Could you check a few things on this model? Use its own coordinates, in mm. Face numbers are marked on the shaded views. A direction names the side the tool comes from. Round coordinates to 2 decimals unless told otherwise and drop trailing zeros. Loops run counter-clockwise (first coordinate to the right, second up) from the corner with the lowest first, then second, coordinate; pieces in that order, holes last. Notation, with made-up numbers: (45.5, 4.25) -> (94.5, 4.25) arc R22 cw to (94.5, 21.25) -> close; hole circle Ø5 at (-20.75, -35). An arc over 180 degrees is marked (long way). One line per item, written item: value.
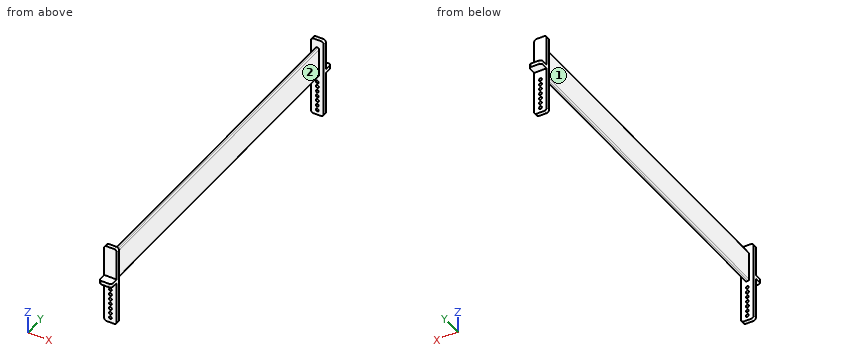
```python
from build123d import *

# Parameters (mm, degrees)
F0_W     = 15.875
F0_H     = 101.6
F4_DEPTH = 4.7625
F2_W     = 15.875
F2_H     = 4.7625
F5_DEPTH = 10.795
F1_W     = 4.7625
F1_H     = 38.1
F6_DEPTH = 431.8
F7_START = 431.8
F7_DEPTH = 4.7625
F8_START = 436.5625
F8_DEPTH = 10.795
F3_R     = 1.905
F3_R_2   = 1.8018515142
F3_R_3   = 1.8092820601
F9_DEPTH = 447.3585
F11_R    = 1.5875
F12_R    = 3.175


with BuildPart() as f4:
    # F0 (on Front) → F4 (new body)
    with BuildSketch(Plane.XZ):
        Rectangle(F0_W, F0_H)
    extrude(amount=F4_DEPTH)

    # F2 (on Front) → F5 (join)
    with BuildSketch(Plane.XZ):
        with Locations((0, 8.28675)):
            Rectangle(F2_W, F2_H)
    extrude(amount=-F5_DEPTH)

    # F1 (on Front) → F6 (join)
    with BuildSketch(Plane.XZ):
        with Locations((0, 21.2725)):
            Rectangle(F1_W, F1_H)
    extrude(amount=F6_DEPTH)

    # F0 (on Front) → F7 (join)
    with BuildSketch(Plane.XZ.offset(F7_START)):
        Rectangle(F0_W, F0_H)
    extrude(amount=F7_DEPTH)

    # F2 (on Front) → F8 (join)
    with BuildSketch(Plane.XZ.offset(F8_START)):
        with Locations((0, 8.28675)):
            Rectangle(F2_W, F2_H)
    extrude(amount=F8_DEPTH)

    # F3 (on Front) → F9 (cut, through all)
    with BuildSketch(Plane.XZ):
        with Locations((0, -31.75)):
            Circle(F3_R)
        with Locations((0, -38.1)):
            Circle(F3_R_2)
        with Locations((0, -44.45)):
            Circle(F3_R_3)
        with Locations((0, -12.7)):
            Circle(F3_R)
        with Locations((0, -19.05)):
            Circle(F3_R_2)
        with Locations((0, -25.4)):
            Circle(F3_R_3)
        with Locations((0, -6.35)):
            Circle(F3_R_2)
    extrude(amount=F9_DEPTH, mode=Mode.SUBTRACT)

    # F11
    f11_edges = [f4.edges().sort_by_distance(p)[0] for p in [
        (-2.38125, -218.28125, 40.3225),
        (2.38125, -218.28125, 40.3225),
        (2.38125, -218.28125, 2.2225),
        (-2.38125, -218.28125, 2.2225),
    ]]
    fillet(f11_edges, radius=F11_R)

    # F12
    f12_edges = [f4.edges().sort_by_distance(p)[0] for p in [
        (7.9375, -434.18125, 50.8),
        (-7.9375, -434.18125, 50.8),
        (7.9375, -434.18125, -50.8),
        (-7.9375, -434.18125, -50.8),
        (-7.9375, -447.3575, 8.28675),
        (7.9375, -447.3575, 8.28675),
        (7.9375, -2.38125, 50.8),
        (-7.9375, -2.38125, 50.8),
        (7.9375, -2.38125, -50.8),
        (-7.9375, -2.38125, -50.8),
        (-7.9375, 10.795, 8.28675),
        (7.9375, 10.795, 8.28675),
    ]]
    fillet(f12_edges, radius=F12_R)


solid = f4.part
```
(1) On a 3-axis mill with a long thin cutter (end or side, diameter ignored), from which of +Z, -Z, +X, -X, +Y, -Y can I reach the whole of each face in a straight line? I mean the marked faces 1 and 2. Say none if no direction works.
Results below:
face 1: +Z, -Z, -X
face 2: +Z, -Z, +X
(2) Please list where these lines run through material, in increasing order: L1, parallel to X at y = -433, z = -44; L2, parallel to Y at x = 4, z = 37; L3, parallel to Y at x = 5.25, z = 6.5.
Results below:
L1: x = -7.94 to -1.75, 1.75 to 7.94
L2: y = -436.56 to -431.8, -4.76 to 0
L3: y = -447.32 to -431.8, -4.76 to 10.76
(3) Imagine slicing it at A-A on y = -144.5. Write out the boundary of the cut face in (x, z) (1 decimal).
Results below:
outline: (-2.4, 3.8) arc R1.6 ccw to (-0.8, 2.2) -> (0.8, 2.2) arc R1.6 ccw to (2.4, 3.8) -> (2.4, 38.7) arc R1.6 ccw to (0.8, 40.3) -> (-0.8, 40.3) arc R1.6 ccw to (-2.4, 38.7) -> close
(4) For pin 1 Ø2 at (x, z) = (0, -6.35) entering from +Y; pin 2 Ø4.5 at (x, z) = (0, -44.45) entering from +Y; pin 3 Ø8 at (y, z) = (-267, 18.5) entering from +X; pin 4 Ø2 at (x, y) = (2, -331.5) entering from +Z, each with a flat end and sliding along its axis, tell me the tip position at first contact or that it passes through.
Results below:
pin 1: passes through
pin 2: stops at y = 0
pin 3: stops at x = 2.38
pin 4: stops at z = 40.31
